```python
from build123d import *

# Parameters (mm, degrees)
BOARDOUTLINE_DEPTH          = 1.6
SKETCH2_R                   = 0.75
SKETCH2_R_2                 = 0.8
COMPONENTHOLES_DEPTH        = 65.998538445
SOLARCELLCONTACTHOLES_DEPTH = 1.6
WINDOWS_1SIDE_DEPTH         = 65.998538445
SKETCH5_W                   = 6
SKETCH5_H                   = 5
CONTACTPADS_DEPTH           = 0.02
M2_CLEARANCE_HOLE1_D        = 2.1
CUT_EXTRUDE1_DEPTH          = 65.999033839
FILLET3_R                   = 1
FILLET3_OF_MIRROR1_R        = 1


with BuildPart() as part:
    # Sketch1 → boardOutline (new body)
    with BuildSketch(Plane.XY):
        with BuildLine():
            Line((-39.5, -50), (39.5, -50))
            ThreePointArc((39.5, -50), (40.914213562, -49.414213562), (41.5, -48))
            Line((41.5, -48), (41.5, 48))
            ThreePointArc((41.5, 48), (40.914213562, 49.414213562), (39.5, 50))
            Line((39.5, 50), (-39.5, 50))
            ThreePointArc((-39.5, 50), (-40.914213562, 49.414213562), (-41.5, 48))
            Line((-41.5, 48), (-41.5, -48))
            ThreePointArc((-41.5, -48), (-40.914213562, -49.414213562), (-39.5, -50))
        make_face()
    extrude(amount=BOARDOUTLINE_DEPTH)

    # Sketch2 → componentHoles (cut, through all)
    with BuildSketch(Plane.XY.offset(1.6)):
        Circle(SKETCH2_R)
        with Locations((-5.385, 42.1)):
            Circle(SKETCH2_R_2)
        with Locations((5.385, 42.1)):
            Circle(SKETCH2_R_2)
    extrude(amount=-COMPONENTHOLES_DEPTH, mode=Mode.SUBTRACT)

    # Sketch4 → solarCellContactHoles (cut)
    with BuildSketch(Plane.XY.offset(1.6)):
        with BuildLine():
            Line((-27.5, 39.25), (-27.5, 45.25))
            ThreePointArc((-27.5, 45.25), (-27, 45.75), (-26.5, 45.25))
            Line((-26.5, 45.25), (-26.5, 39.25))
            ThreePointArc((-26.5, 39.25), (-27, 38.75), (-27.5, 39.25))
        make_face()
        with BuildLine():
            Line((26.5, 39.25), (26.5, 45.25))
            ThreePointArc((26.5, 45.25), (27, 45.75), (27.5, 45.25))
            Line((27.5, 45.25), (27.5, 39.25))
            ThreePointArc((27.5, 39.25), (27, 38.75), (26.5, 39.25))
        make_face()
        with BuildLine():
            Line((26.5, -46.25), (26.5, -40.25))
            ThreePointArc((26.5, -40.25), (27, -39.75), (27.5, -40.25))
            Line((27.5, -40.25), (27.5, -46.25))
            ThreePointArc((27.5, -46.25), (27, -46.75), (26.5, -46.25))
        make_face()
        with BuildLine():
            Line((-27.5, -46.25), (-27.5, -40.25))
            ThreePointArc((-27.5, -40.25), (-27, -39.75), (-26.5, -40.25))
            Line((-26.5, -40.25), (-26.5, -46.25))
            ThreePointArc((-26.5, -46.25), (-27, -46.75), (-27.5, -46.25))
        make_face()
    extrude(amount=-SOLARCELLCONTACTHOLES_DEPTH, mode=Mode.SUBTRACT)

    # Sketch3 → windows_1side (cut, through all)
    with BuildSketch(Plane.XY.offset(1.6)):
        with BuildLine():
            Line((-35.5, 37), (-29, 37))
            ThreePointArc((-29, 37), (-27.585786438, 36.414213562), (-27, 35))
            Line((-27, 35), (-27, 23))
            ThreePointArc((-27, 23), (-27.585786438, 21.585786438), (-29, 21))
            Line((-29, 21), (-35.5, 21))
            ThreePointArc((-35.5, 21), (-36.914213562, 21.585786438), (-37.5, 23))
            Line((-37.5, 23), (-37.5, 35))
            ThreePointArc((-37.5, 35), (-36.914213562, 36.414213562), (-35.5, 37))
        make_face()
        with BuildLine():
            Line((-29, -22), (-35.5, -22))
            ThreePointArc((-35.5, -22), (-36.914213562, -22.585786438), (-37.5, -24))
            Line((-37.5, -24), (-37.5, -35))
            ThreePointArc((-37.5, -35), (-36.914213562, -36.414213562), (-35.5, -37))
            Line((-35.5, -37), (-29, -37))
            ThreePointArc((-29, -37), (-27.585786438, -36.414213562), (-27, -35))
            Line((-27, -35), (-27, -24))
            ThreePointArc((-27, -24), (-27.585786438, -22.585786438), (-29, -22))
        make_face()
        with BuildLine():
            Line((-29, -19), (-35.5, -19))
            ThreePointArc((-35.5, -19), (-36.914213562, -18.414213562), (-37.5, -17))
            Line((-37.5, -17), (-37.5, 16))
            ThreePointArc((-37.5, 16), (-36.914213562, 17.414213562), (-35.5, 18))
            Line((-35.5, 18), (-29, 18))
            ThreePointArc((-29, 18), (-27.585786438, 17.414213562), (-27, 16))
            Line((-27, 16), (-27, -17))
            ThreePointArc((-27, -17), (-27.585786438, -18.414213562), (-29, -19))
        make_face()
    windows_1side = extrude(amount=-WINDOWS_1SIDE_DEPTH, mode=Mode.SUBTRACT)

    # Sketch5 → contactPads (add)
    with BuildSketch(Plane.XY.offset(1.6)):
        with Locations((-22.5, 35)):
            Rectangle(SKETCH5_W, SKETCH5_H)
        with Locations((22.5, 35)):
            Rectangle(SKETCH5_W, SKETCH5_H)
        with Locations((22.5, -36)):
            Rectangle(SKETCH5_W, SKETCH5_H)
        with Locations((-22.5, -36)):
            Rectangle(SKETCH5_W, SKETCH5_H)
    extrude(amount=CONTACTPADS_DEPTH)

    # M2 Clearance Hole1 (through all)
    with Locations(Plane(origin=(0, 0, 0), x_dir=(-1, 0, 0), z_dir=(0, 0, -1))):
        with Locations((39.5, 45), (39.5, -15), (39.5, -45), (39.5, 15)):
            m2_clearance_hole1 = Hole(M2_CLEARANCE_HOLE1_D / 2)

    # Sketch10 → Cut-Extrude1 (cut, symmetric)
    with BuildSketch(Plane(origin=(0, 0, 0), x_dir=(-1, 0, 0), z_dir=(0, 0, -1))):
        with BuildLine():
            Line((15.45, 48), (15.45, 55.073166109))
            ThreePointArc((15.45, 55.073166109), (16.5, 56.123166109), (17.55, 55.073166109))
            Line((17.55, 55.073166109), (17.55, 48))
            ThreePointArc((17.55, 48), (16.5, 46.95), (15.45, 48))
        make_face()
        with BuildLine():
            Line((17.55, -48.5), (17.55, -55.573166109))
            ThreePointArc((17.55, -55.573166109), (16.5, -56.623166109), (15.45, -55.573166109))
            Line((15.45, -55.573166109), (15.45, -48.5))
            ThreePointArc((15.45, -48.5), (16.5, -47.45), (17.55, -48.5))
        make_face()
    cut_extrude1 = extrude(amount=CUT_EXTRUDE1_DEPTH, both=True, mode=Mode.SUBTRACT)

    # Fillet3
    fillet3_edges = [part.edges().sort_by_distance(p)[0] for p in [
        (-15.45, 50, 0.8),
        (-17.55, 50, 0.8),
        (-17.55, -50, 0.8),
        (-15.45, -50, 0.8),
    ]]
    fillet(fillet3_edges, radius=FILLET3_R)

    # Mirror1: windows_1side, M2 Clearance Hole1, Cut-Extrude1 across plane
    add(windows_1side.mirror(Plane(origin=(0, 0, 0), x_dir=(0, 0, 1), z_dir=(1, 0, 0))), mode=Mode.SUBTRACT)
    add(m2_clearance_hole1.mirror(Plane(origin=(0, 0, 0), x_dir=(0, 0, 1), z_dir=(1, 0, 0))), mode=Mode.SUBTRACT)
    add(cut_extrude1.mirror(Plane(origin=(0, 0, 0), x_dir=(0, 0, 1), z_dir=(1, 0, 0))), mode=Mode.SUBTRACT)

    # Fillet3 of Mirror1
    fillet3_of_mirror1_edges = [part.edges().sort_by_distance(p)[0] for p in [
        (15.45, 50, 0.8),
        (17.55, 50, 0.8),
        (17.55, -50, 0.8),
        (15.45, -50, 0.8),
    ]]
    fillet(fillet3_of_mirror1_edges, radius=FILLET3_OF_MIRROR1_R)


solid = part.part
```
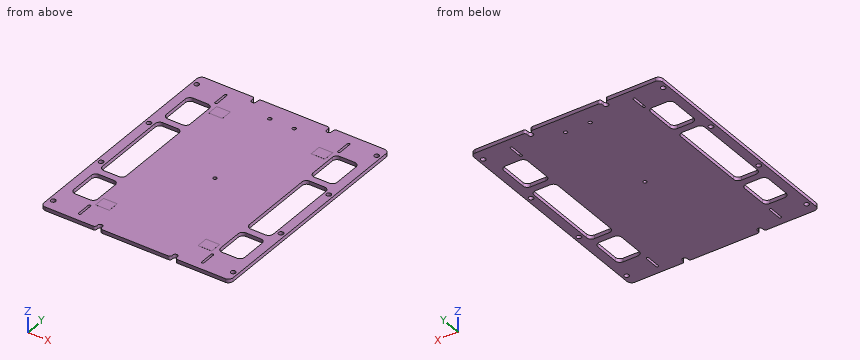
CAD build for the part. Positions are in the model's coordinates, mm. Coordinates: 2 decimals unless noted, no trailing zeros. Order: outer loops, then holes, each group sorted by start corner. A loop starts at its lowest first (then second) coordinate and runs counter-clockwise, first axis right, second up. Notation, with made-up numbers: (55, 3.25) - (101, 3.25) arc R26 cw to (101, 34.25) - close; hole circle Ø4 at (70, 12.5). An arc over 180 degrees is marked (long way). Answer in a Markdown table with one row per item.
1. Slice it at A-A, the plane y = -26.5. List the corners of the cut face in (x, z).
Answer:
| item | result |
|---|---|
| outline | (-41.5, 0) - (-37.5, 0) - (-37.5, 1.6) - (-41.5, 1.6) - close; (-27, 0) - (27, 0) - (27, 1.6) - (-27, 1.6) - close; (37.5, 0) - (41.5, 0) - (41.5, 1.6) - (37.5, 1.6) - close |
2. Slice it at B-B, the plane y = -15. List the corners of the cut face in (x, z).
Answer:
| item | result |
|---|---|
| outline | (-41.5, 0) - (-40.55, 0) - (-40.55, 1.6) - (-41.5, 1.6) - close; (-38.45, 0) - (-37.5, 0) - (-37.5, 1.6) - (-38.45, 1.6) - close; (-27, 0) - (27, 0) - (27, 1.6) - (-27, 1.6) - close; (37.5, 0) - (38.45, 0) - (38.45, 1.6) - (37.5, 1.6) - close; (40.55, 0) - (41.5, 0) - (41.5, 1.6) - (40.55, 1.6) - close |
3. Flat gauge pins, fed straight in: P1, Ø0.5, axis at y = 48.5, z = 1, coming from the +X side; P2, Ø3.5, axis at x = 39.5, y = -15, coming from the +Z side; P3, Ø1.7, axis at x = -39.5, y = -45, coming from the -Z side. Where does each tip first touch, or does it go through?
Answer:
| item | result |
|---|---|
| P1 | x = 41.48 |
| P2 | z = 1.6 |
| P3 | through |
4. Slice it at D-D, the plane y = -45. List the corners of the cut face in (x, z), then the cut area to 3 significant figures.
Answer:
| item | result |
|---|---|
| outline | (-41.5, 0) - (-40.55, 0) - (-40.55, 1.6) - (-41.5, 1.6) - close; (-38.45, 0) - (-27.5, 0) - (-27.5, 1.6) - (-38.45, 1.6) - close; (-26.5, 0) - (26.5, 0) - (26.5, 1.6) - (-26.5, 1.6) - close; (27.5, 0) - (38.45, 0) - (38.45, 1.6) - (27.5, 1.6) - close; (40.55, 0) - (41.5, 0) - (41.5, 1.6) - (40.55, 1.6) - close |
| area | 123 mm² |
5. Slice it at C-C, the plane z = 0.6. Give the number of separate pieces and of enclosed holes in the cut face, then the cut area to 3 significant figures.
Answer:
| item | result |
|---|---|
| separate pieces | 1 |
| enclosed holes | 21 |
| area | 6,810 mm² |
6. Drill centre lines: L1, parallel to X at y = 40, z = 1.05; L2, parallel to X at y = 42.1, z = 1.25 (3 decimals); L3, parallel to X at y = -28, z = 0.25. Where is each one in solid material? Low to high. Write a range as from..to.
Answer:
| item | result |
|---|---|
| L1 | -41.5..-27.5, -26.5..26.5, 27.5..41.5 |
| L2 | -41.5..-27.5, -26.5..-6.185, -4.585..4.585, 6.185..26.5, 27.5..41.5 |
| L3 | -41.5..-37.5, -27..27, 37.5..41.5 |
